```python
from build123d import *

# Parameters (mm, degrees)
F0_W     = 800
F0_H     = 600
F0_W_2   = 30
F0_H_2   = 400
F1_DEPTH = 50


with BuildPart() as f1:
    # F0 (on Front) → F1 (new body, symmetric)
    with BuildSketch(Plane.XZ):
        with Locations((400, 250)):
            Rectangle(F0_W, F0_H)
        with Locations((80, 250)):
            Rectangle(F0_W_2, F0_H_2, mode=Mode.SUBTRACT)
        with Locations((160, 250)):
            Rectangle(F0_W_2, F0_H_2, mode=Mode.SUBTRACT)
        with Locations((240, 250)):
            Rectangle(F0_W_2, F0_H_2, mode=Mode.SUBTRACT)
        with Locations((320, 250)):
            Rectangle(F0_W_2, F0_H_2, mode=Mode.SUBTRACT)
        with Locations((400, 250)):
            Rectangle(F0_W_2, F0_H_2, mode=Mode.SUBTRACT)
        with Locations((480, 250)):
            Rectangle(F0_W_2, F0_H_2, mode=Mode.SUBTRACT)
        with Locations((560, 250)):
            Rectangle(F0_W_2, F0_H_2, mode=Mode.SUBTRACT)
        with Locations((640, 250)):
            Rectangle(F0_W_2, F0_H_2, mode=Mode.SUBTRACT)
        with Locations((720, 250)):
            Rectangle(F0_W_2, F0_H_2, mode=Mode.SUBTRACT)
    extrude(amount=F1_DEPTH, both=True)


solid = f1.part
```
For this review, take the finished solid that the model builds, in its own axes (mm). A direction names the side the tool comes from. Coordinates: 2 decimals unless noted, no trailing zeros.
(1) Wall thickness on probe 1 along Z at (x, y) = (393, -33): over which ranges is the line inside the solid? List them lowest first.
(2) Add section A-A on y = -41. Count the separate pieces of the cut face and the enclosed holes in it, then the cut area to 3 significant figures.
(3) The part is to be moulded in two halves that separate along X. For faces 1 (the face through (800, -1, 246)), 2 (the face through (575, -1, 247)), 3 (the face through (394, -1, -50)), say which applies: +X half, -X half, draft (parallel to the pull), parting line (faces both ways), or undercut.
(4) Tool access review of faces 4 (the face through (80, -1, 450)), 5 (the face through (394, -1, 550)): name each direction out of +Z, -Z, +X, -X, +Y, -Y from which nothing blocks a thin tool from reaching the whole face with its end or side.
Answer sheet:
1. probe 1: z = -50 to 50, 450 to 550
2. separate pieces: 1
2. enclosed holes: 9
2. area: 372,000 mm2
3. face 1: +X half
3. face 2: undercut
3. face 3: draft
4. face 4: +Y, -Y
4. face 5: +Z, +X, -X, +Y, -Y
